from build123d import *

# Parameters (mm, degrees)
SKETCH_1_R      = 1.6
EXTRUDE_1_DEPTH = 2
SKETCH_2_W      = 25
SKETCH_2_H      = 50
EXTRUDE_2_DEPTH = 13.75
SKETCH_3_R      = 12.5
EXTRUDE_3_DEPTH = 10.25


with BuildPart() as part:
    # 草图1 → 凸台-拉伸1 (new body)
    with BuildSketch(Plane(origin=(0, 0, 0), x_dir=(1, 0, 0), z_dir=(0, 1, 0))):
        Polygon((-12.5, 25), (12.5, 25), (12.5, 17.760130657), (17.680206778, 17.760130657), (17.680206778, 12.943452398), (12.5, 12.943452398), (12.5, -12.943452398), (17.680206778, -12.943452398), (17.680206778, -17.760130657), (12.5, -17.760130657), (12.5, -25), (-12.5, -25), (-12.5, -17.760130657), (-17.680206778, -17.760130657), (-17.680206778, -12.943452398), (-12.5, -12.943452398), (-12.5, 12.943452398), (-17.680206778, 12.943452398), (-17.680206778, 17.760130657), (-12.5, 17.760130657), align=None)
        with Locations(Location((15.25, 15.25, 0), (0, 0, 270))):
            Circle(SKETCH_1_R, mode=Mode.SUBTRACT)
        with Locations(Location((-15.25, 15.25, 0), (0, 0, 90))):
            Circle(SKETCH_1_R, mode=Mode.SUBTRACT)
        with Locations(Location((15.25, -15.25, 0), (0, 0, 90))):
            Circle(SKETCH_1_R, mode=Mode.SUBTRACT)
        with Locations(Location((-15.25, -15.25, 0), (0, 0, 270))):
            Circle(SKETCH_1_R, mode=Mode.SUBTRACT)
    extrude(amount=EXTRUDE_1_DEPTH)

    # 草图2 → 凸台-拉伸2 (add)
    with BuildSketch(Plane(origin=(0, 2, 0), x_dir=(1, 0, 0), z_dir=(0, 1, 0))):
        Rectangle(SKETCH_2_W, SKETCH_2_H)
    extrude(amount=EXTRUDE_2_DEPTH)

    # 草图3 → 凸台-拉伸3 (add)
    with BuildSketch(Plane.XZ):
        with Locations(Location((0, 12.5, 0), (0, 0, 90))):
            Circle(SKETCH_3_R)
    extrude(amount=EXTRUDE_3_DEPTH)


solid = part.part
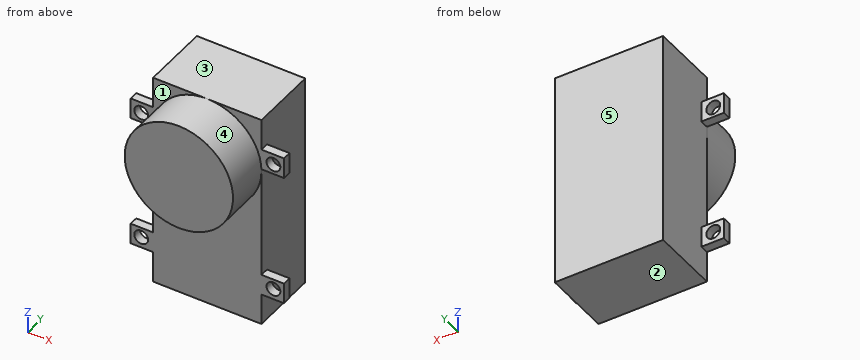
Build history of the part. All positions in model axes, mm. Face numbers are marked on the shaded views. A direction names the side the tool comes from. Round coordinates to 2 decimals unless told otherwise and drop trailing zeros. Loops run counter-clockwise (first coordinate to the right, second up) from the corner with the lowest first, then second, coordinate; pieces in that order, holes last. Notation, with made-up numbers: (-11, 10) -> (19, 10) arc R19 ccw to (19, 27) -> close; hole circle Ø11 at (31.5, -2.75). An arc over 180 degrees is marked (long way). Use CSV: the item, a comma, the result in double quotes. Start each with the question number.
Q1. Drill centre lines: L1, parallel to X at y = 1.55, z = -15.25; L2, parallel to X at y = 11.75, z = -8.5; L3, parallel to Y at x = 0, z = -1. Where is each one in solid material? Low to high.
Q2. Which spindle directions (+Z, -Z, +X, -X, +Y, -Y) get a long thin tool onto all of the face, cutting with end or side? Do the marked faces 1 and 2. Say none if no direction does.
Q3. Saw through at A-A on z = -15.25. Give the cut face in (x, y), and give its area (3 significant figures).
Q4. Flat gauge pins, fed straight in: pin 1 Ø4 at (y, z) = (6.5, 5) entering from +X; pin 2 Ø1.5 at (y, z) = (6.5, 1) entering from -X; pin 3 Ø1.6 at (x, y) = (-14, 1) entering from -Z. Where does each tip first touch, or does it go through?
Q5. Saw through at B-B on x = 15.25. Give the cut face in (y, z), and give its area (3 significant figures).
Q6. Saw through at C-C on x = -1.5. Give the cut face in (y, z).
Q7. Saw through at D-D on z = 4. Give the cut face in (x, y), and give its area (3 significant figures).
Q8. Mould opens along Z. For the marked faces 3, 4 and 5 say: +Z half, -Z half, draft (parallel to the pull), parting line (faces both ways), or undercut.
Solutions:
1,L1,"x = -17.68 to -16.85, -13.65 to 13.65, 16.85 to 17.68"
1,L2,"x = -12.5 to 12.5"
1,L3,"y = 0 to 15.75"
2,face 1,"+Z, -X, -Y"
2,face 2,"-Z, +X, -X, +Y, -Y"
3,outline,"(-17.68, 0) -> (-16.85, 0) -> (-16.85, 2) -> (-17.68, 2) -> close; (-13.65, 0) -> (13.65, 0) -> (13.65, 2) -> (12.5, 2) -> (12.5, 15.75) -> (-12.5, 15.75) -> (-12.5, 2) -> (-13.65, 2) -> close; (16.85, 0) -> (17.68, 0) -> (17.68, 2) -> (16.85, 2) -> close"
3,area,"402 mm^2"
4,pin 1,"stops at x = 12.5"
4,pin 2,"stops at x = -12.5"
4,pin 3,"stops at z = -17.76"
5,outline,"(0, -17.76) -> (2, -17.76) -> (2, -16.85) -> (0, -16.85) -> close; (0, -13.65) -> (2, -13.65) -> (2, -12.94) -> (0, -12.94) -> close; (0, 12.94) -> (2, 12.94) -> (2, 13.65) -> (0, 13.65) -> close; (0, 16.85) -> (2, 16.85) -> (2, 17.76) -> (0, 17.76) -> close"
5,area,"6.47 mm^2"
6,outline,"(-10.25, 0.09) -> (0, 0.09) -> (0, -25) -> (15.75, -25) -> (15.75, 25) -> (0, 25) -> (0, 24.91) -> (-10.25, 24.91) -> close"
7,outline,"(-12.5, 0) -> (-9.17, 0) -> (-9.17, -10.25) -> (9.17, -10.25) -> (9.17, 0) -> (12.5, 0) -> (12.5, 15.75) -> (-12.5, 15.75) -> close"
7,area,"582 mm^2"
8,face 3,"+Z half"
8,face 4,"parting line"
8,face 5,"draft"
